```python
from build123d import *

# Parameters (mm, degrees)
SALIENTE_EXTRUIR1_DEPTH = 3
CROQUIS4_W              = 15
CROQUIS4_H              = 6
CROQUIS4_W_2            = 10
CROQUIS4_H_2            = 3
CORTAR_EXTRUIR1_DEPTH   = 3
SALIENTE_EXTRUIR2_DEPTH = 3
REDONDEO1_R             = 1
REDONDEO2_R             = 0.25


with BuildPart() as part:
    # Croquis3 → Saliente-Extruir1 (new body)
    with BuildSketch(Plane(origin=(0, 0, 0), x_dir=(1, 0, 0), z_dir=(0, 1, 0))):
        with BuildLine():
            Line((-50, -45), (50, -45))
            Line((50, -45), (50, -40.05))
            Line((50, -40.05), (53, -40.05))
            Line((53, -40.05), (53, -35.05))
            Line((53, -35.05), (56, -35.05))
            Line((56, -35.05), (56, -40.05))
            Line((56, -40.05), (59, -40.05))
            Line((59, -40.05), (59, -32.55))
            ThreePointArc((59, -32.55), (58.267766953, -30.782233047), (56.5, -30.05))
            Line((56.5, -30.05), (50, -30.05))
            Line((50, -30.05), (50, 28.189923373))
            Line((50, 28.189923373), (50.1, 38.189923373))
            Line((50.1, 38.189923373), (50.1, 43.139923373))
            ThreePointArc((50.1, 43.139923373), (49.605586306, 44.632445926), (48.317901143, 45.534629607))
            Line((48.317901143, 45.534629607), (0.615531773, 59.835166775))
            ThreePointArc((0.615531773, 59.835166775), (0, 59.908733938), (-0.615531773, 59.835166775))
            Line((-0.615531773, 59.835166775), (-48.317901143, 45.534629607))
            ThreePointArc((-48.317901143, 45.534629607), (-49.605586306, 44.632445926), (-50.1, 43.139923373))
            Line((-50.1, 43.139923373), (-50.1, 38.189923373))
            Line((-50.1, 38.189923373), (-50, 28.189923373))
            Line((-50, 28.189923373), (-50, -30.05))
            Line((-50, -30.05), (-56.5, -30.05))
            ThreePointArc((-56.5, -30.05), (-58.267766953, -30.782233047), (-59, -32.55))
            Line((-59, -32.55), (-59, -40.05))
            Line((-59, -40.05), (-56, -40.05))
            Line((-56, -40.05), (-56, -35.05))
            Line((-56, -35.05), (-53, -35.05))
            Line((-53, -35.05), (-53, -40.05))
            Line((-53, -40.05), (-50, -40.05))
            Line((-50, -40.05), (-50, -45))
        make_face()
        Polygon((-23.595339952, 49.778243466), (-18.595339952, 51.277177099), (-17.695979772, 48.277177099), (-27.695979772, 45.279309832), (-28.595339952, 48.279309832), align=None, mode=Mode.SUBTRACT)
        Polygon((28.595339952, 48.279309832), (27.695979772, 45.279309832), (17.695979772, 48.277177099), (18.595339952, 51.277177099), (23.595339952, 49.778243466), align=None, mode=Mode.SUBTRACT)
    extrude(amount=SALIENTE_EXTRUIR1_DEPTH)

    # Croquis4 → Cortar-Extruir1 (cut, symmetric)
    with BuildSketch(Plane(origin=(0, 3, 0), x_dir=(1, 0, 0), z_dir=(0, 1, 0))):
        with Locations((0, -39)):
            Rectangle(CROQUIS4_W, CROQUIS4_H)
        with Locations((-33, -43.5)):
            Rectangle(CROQUIS4_W_2, CROQUIS4_H_2)
        with Locations((33, -43.5)):
            Rectangle(CROQUIS4_W_2, CROQUIS4_H_2)
        with Locations((0, -28.5)):
            Rectangle(CROQUIS4_W, CROQUIS4_H_2)
    extrude(amount=CORTAR_EXTRUIR1_DEPTH, both=True, mode=Mode.SUBTRACT)

    # Croquis5 → Saliente-Extruir2 (add)
    with BuildSketch(Plane(origin=(0, 0, 0), x_dir=(1, 0, 0), z_dir=(0, 1, 0))):
        with BuildLine():
            Line((-50, -45), (50, -45))
            Line((50, -45), (50, -45.5))
            ThreePointArc((50, -45.5), (49.267766953, -47.267766953), (47.5, -48))
            Line((47.5, -48), (-47.5, -48))
            ThreePointArc((-47.5, -48), (-49.267766953, -47.267766953), (-50, -45.5))
            Line((-50, -45.5), (-50, -45))
        make_face()
    extrude(amount=SALIENTE_EXTRUIR2_DEPTH)

    # Redondeo1
    redondeo1_edges = [part.edges().sort_by_distance(p)[0] for p in [
        (-59, 1.5, 40.05),
        (59, 1.5, 40.05),
    ]]
    fillet(redondeo1_edges, radius=REDONDEO1_R)

    # Redondeo2
    redondeo2_edges = [part.edges().sort_by_distance(p)[0] for p in [
        (-50, 1.5, 40.05),
        (-53, 1.5, 40.05),
        (-53, 1.5, 35.05),
        (-56, 1.5, 35.05),
        (-56, 1.5, 40.05),
        (-50, 1.5, 30.05),
        (50, 1.5, 30.05),
        (56, 1.5, 40.05),
        (56, 1.5, 35.05),
        (53, 1.5, 35.05),
        (53, 1.5, 40.05),
        (50, 1.5, 40.05),
    ]]
    fillet(redondeo2_edges, radius=REDONDEO2_R)


solid = part.part
```
Geometry check sheet. Reference: the model listing, model coordinates, mm. A direction names the side the tool comes from. Round coordinates to 2 decimals unless told otherwise and drop trailing zeros. Loops run counter-clockwise (first coordinate to the right, second up) from the corner with the lowest first, then second, coordinate; pieces in that order, holes last. Notation, with made-up numbers: M 78,-38.75 L 125,-38.75 A5 ccw 125,-34.75 Z; hole C -23.5,45 d7. An arc over 180 degrees is marked long. Return JSON: item names as keys, results as strings. Group by question number.
(1) Go/stop test with flat-tipped pins: pin 1 (0.9 mm diameter, centred on y = 1.5, z = 43, fed in from +X); pin 2 (1.2 mm diameter, centred on x = -52, y = 1, fed in from +Z); pin 3 (6 mm diameter, centred on x = -4.5, z = 15, fed in from -Y). Record where each tip stops, or that it passes through.
(2) Mould release check, pull along Z, two halves, no side actions. Record for faces 4 (the face through (54, 1, 35.05)), 5 (the face through (-28.14, 1.48, -46.76)), 6 (the face through (-53, 1, 38)): pulls with the +Z half, pulls with the -Z half, needs draft (parallel to the pull), parting line crosses it, or undercut.
(3) Set-up check for faces 1 (the face through (-50, 1, 43)), 2 (the face through (56, 1, 38)), 3 (the face through (-38, 1, 44)): record each of +Z, -Z, +X, -X, +Y, -Y from which the full face is reachable in a straight line by a thin tool's end or side.
(4) Scan lines: line 1 along Z through (x, y) = (0.5, 0.85); line 2 along X through (y, z) = (0.25, 28); line 3 along X through (y, z) = (0.25, 23.5). Record each from-to range of solid material in increasing order. Write a range as [from, to].
(5) Section check C-C, the plane y = 0.9. Give the number of separate pieces and of enclosed holes in the cut face, and give its area (3 significant figures).
(6) Section check A-A, the plane x = 31. Enter the section's corners in (y, z), and give its area (3 significant figures).
(7) Section check D-D, the plane x = -32.5. Enter the section's corners in (y, z), and give its area (3 significant figures).
(8) Section check B-B, the plane z = 12. Enter the section's corners in (x, y).
Data:
{
 "1": {"pin 1": "x = 50", "pin 2": "z = 40.05", "pin 3": "y = 0"},
 "2": {"face 4": "pulls with the +Z half", "face 5": "undercut", "face 6": "needs draft"},
 "3": {"face 1": "+Z, -X, +Y, -Y", "face 2": "+Z, +Y, -Y", "face 3": "+Y, -Y"},
 "4": {"line 1": "[-59.86, 27], [30, 36], [42, 48]", "line 2": "[-50, -7.5], [7.5, 50]", "line 3": "[-50, 50]"},
 "5": {"separate pieces": "1", "enclosed holes": "6", "area": "9,940 mm²"},
 "6": {"outline": "M 0,-50.73 L 3,-50.73 L 3,42 L 0,42 Z; M 0,45 L 3,45 L 3,48 L 0,48 Z", "area": "287 mm²"},
 "7": {"outline": "M 0,-50.28 L 3,-50.28 L 3,42 L 0,42 Z; M 0,45 L 3,45 L 3,48 L 0,48 Z", "area": "286 mm²"},
 "8": {"outline": "M -50,0 L 50,0 L 50,3 L -50,3 Z"}
}
